Could you check a few things on this model? Use its own coordinates, in mm. Give positions to 0.01 mm unless a question says otherwise; leave off trailing zeros. Write each loop counter-clockwise with the first axis right and the second up, starting at its lowest first coordinate (ties: lowest second). Pieces come first, ordered by that corner, then holes. Notation, with made-up numbers: (25, 86) - (58, 86) arc R8 cw to (58, 91) - close; hole circle Ø10 at (-36, 11). An arc over 180 degrees is marked (long way). Write item = value, one per line.
from build123d import *

# Parameters (mm, degrees)
SKETCH_W        = 20
SKETCH_H        = 20
PAD_DEPTH       = 50
SKETCH001_R     = 4.1
POCKET_DEPTH    = 20
SKETCH002_R     = 4.1
POCKET001_DEPTH = 20


with BuildPart() as part:
    # Sketch → Pad (new body)
    with BuildSketch(Plane.XY):
        with Locations((-14.537711, 19.886208)):
            Rectangle(SKETCH_W, SKETCH_H)
    extrude(amount=PAD_DEPTH)

    # Sketch001 → Pocket (cut)
    with BuildSketch(Plane.YZ.offset(-4.537711)):
        with Locations((19.886208, 30)):
            Circle(SKETCH001_R)
        with Locations((19.886208, 10)):
            Circle(SKETCH001_R)
    extrude(amount=-POCKET_DEPTH, mode=Mode.SUBTRACT)

    # Sketch002 → Pocket001 (cut)
    with BuildSketch(Plane.XZ.offset(-9.886208)):
        with Locations((-14.537711, 46)):
            Circle(SKETCH002_R)
    extrude(amount=-POCKET001_DEPTH, mode=Mode.SUBTRACT)


solid = part.part
1. If we section it at B-B, the plane x = -13: Please give me the cut outline in (y, z).
Filled sheet:
outline = (9.89, 0) - (29.89, 0) - (29.89, 42.2) - (9.89, 42.2) - close; (9.89, 49.8) - (29.89, 49.8) - (29.89, 50) - (9.89, 50) - close; hole circle Ø8.2 at (19.89, 10); hole circle Ø8.2 at (19.89, 30)
2. I need wall thicknesses on line 1 (X direction, y = 24.5, z = 46); line 2 (Z direction, x = -16.75, y = 16.75); line 3 (Z direction, x = -8.25, y = 19). Which ranges of each line are inside material? Lowest first, please.
Filled sheet:
line_1 = -24.54 to -18.64, -10.44 to -4.54
line_2 = 0 to 7.36, 12.64 to 27.36, 32.64 to 42.55, 49.45 to 50
line_3 = 0 to 6, 14 to 26, 34 to 50
3. If we section it at A-A, the plane z = 30: Please give me the cut outline in (x, y), and give its area (3 significant figures).
Filled sheet:
outline = (-24.54, 9.89) - (-4.54, 9.89) - (-4.54, 15.79) - (-24.54, 15.79) - close; (-24.54, 23.99) - (-4.54, 23.99) - (-4.54, 29.89) - (-24.54, 29.89) - close
area = 236 mm2
4. If we section it at C-C, the plane y = 13: Please give me the cut outline in (x, z).
Filled sheet:
outline = (-24.54, 0) - (-4.54, 0) - (-4.54, 50) - (-13.64, 50) arc R4.1 cw (long way) to (-15.44, 50) - (-24.54, 50) - close
5. Thinking about a two-plate mould opening in Z: for faces 1 (the face through (-9, 20, 50)), 2 (the face through (-14.398, 23.797, 11.232)), 3 (the face through (-24.538, 20, 25)), which applies, pulls with the +Z half, pulls with the -Z half, needs draft (parallel to the pull), parting line crosses it, or undercut?
Filled sheet:
face_1 = pulls with the +Z half
face_2 = undercut
face_3 = needs draft
6. If we section it at D-D, the plane x = -21: Please give me the cut outline in (y, z).
Filled sheet:
outline = (9.89, 0) - (29.89, 0) - (29.89, 50) - (9.89, 50) - close; hole circle Ø8.2 at (19.89, 10); hole circle Ø8.2 at (19.89, 30)
7. For pin 1 (6.5 mm diameter, centred on x = -14.54, z = 46, fed in from +Y), with a flat end and sliding along its axis, tell me the tip position at first contact or that it passes through.
Filled sheet:
pin_1 = through
